Model file for the job. Use its own axes, mm. Give positions to 0.01 mm unless a question says otherwise; leave off trailing zeros. Write each loop counter-clockwise with the first axis right and the second up, starting at its lowest first coordinate (ties: lowest second). Pieces come first, ordered by that corner, then holes. Notation, with made-up numbers: (-35, 37) - (-28, 37) arc R22 ccw to (-28, 71) - close; hole circle Ø11 at (87, 53.25). An arc over 180 degrees is marked (long way). Use a Markdown table: item, result. Add a question column.
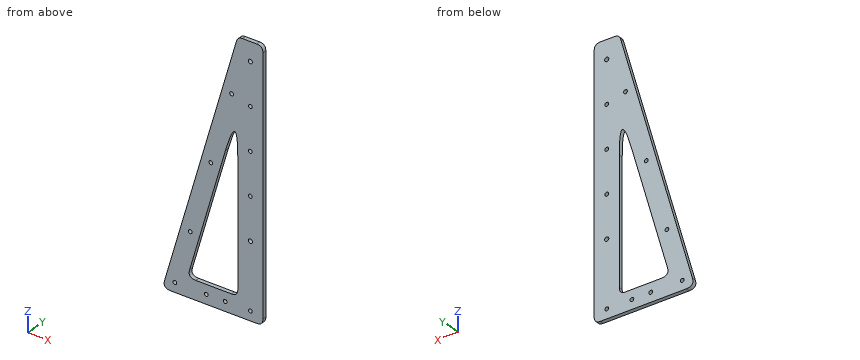
```python
from build123d import *

# Parameters (mm, degrees)
SKETCH1_R           = 1.5
SKETCH1_R_2         = 1.65
BOSS_EXTRUDE1_DEPTH = 3.175
FILLET1_SIZE        = 5


with BuildPart() as part:
    # Sketch1 → Boss-Extrude1 (new body)
    with BuildSketch(Plane(origin=(0, 0, 0), x_dir=(1, 0, 0), z_dir=(0, 1, 0))):
        Polygon((-20, -210), (0, -210), (0, 0), (-80, 0), align=None)
        with Locations(Location((-41.422797756, -107.71979577, 0), (0, 0, 270))):
            Circle(SKETCH1_R, mode=Mode.SUBTRACT)
        with Locations(Location((-24.939530082, -165.411232629, 0), (0, 0, 270))):
            Circle(SKETCH1_R, mode=Mode.SUBTRACT)
        with Locations(Location((-10, -195, 0), (0, 0, 270))):
            Circle(SKETCH1_R_2, mode=Mode.SUBTRACT)
        with BuildLine():
            ThreePointArc((-10, -159.75), (-8.5, -161.25), (-10, -162.75))
            ThreePointArc((-10, -162.75), (-11.5, -161.25), (-10, -159.75))
        make_face(mode=Mode.SUBTRACT)
        with BuildLine():
            ThreePointArc((-10, -126), (-8.5, -127.5), (-10, -129))
            ThreePointArc((-10, -129), (-11.5, -127.5), (-10, -126))
        make_face(mode=Mode.SUBTRACT)
        Polygon((-20, -15), (-20, -155.39917583), (-60.114050237, -15), align=None, mode=Mode.SUBTRACT)
        with Locations(Location((-57.90606543, -50.028358912, 0), (0, 0, 270))):
            Circle(SKETCH1_R, mode=Mode.SUBTRACT)
        with Locations(Location((-70.057025119, -7.5, 0), (0, 0, 270))):
            Circle(SKETCH1_R, mode=Mode.SUBTRACT)
        with Locations(Location((-45.028512559, -7.5, 0), (0, 0, 270))):
            Circle(SKETCH1_R, mode=Mode.SUBTRACT)
        with BuildLine():
            ThreePointArc((-10, -92.25), (-8.5, -93.75), (-10, -95.25))
            ThreePointArc((-10, -95.25), (-11.5, -93.75), (-10, -92.25))
        make_face(mode=Mode.SUBTRACT)
        with Locations(Location((-10, -60, 0), (0, 0, 270))):
            Circle(SKETCH1_R_2, mode=Mode.SUBTRACT)
        with Locations(Location((-30, -7.5, 0), (0, 0, 270))):
            Circle(SKETCH1_R, mode=Mode.SUBTRACT)
        with Locations(Location((-10, -7.5, 0), (0, 0, 270))):
            Circle(SKETCH1_R, mode=Mode.SUBTRACT)
    extrude(amount=BOSS_EXTRUDE1_DEPTH)

    # Fillet1
    # a fillet whose section is not a circle: 5 mm, written as the material it adds along each edge
    with BuildSketch(Plane(origin=(-20, 0, 15), x_dir=(0, 0, 1), z_dir=(0, 1, 0))) as fillet1_piece_1:
        with BuildLine():
            Bezier((FILLET1_SIZE, 0), (0, 0), (0, -FILLET1_SIZE), weights=[1, 1, 1])
            Line((0, -FILLET1_SIZE), (0, 0))
            Line((0, 0), (FILLET1_SIZE, 0))
        make_face()
    extrude(amount=3.175)
    with BuildSketch(Plane(origin=(-60.114050237, 0, 15), x_dir=(0.2747211278973786, 0, 0.9615239476408229), z_dir=(0, 1, 0))) as fillet1_piece_2:
        with BuildLine():
            Bezier((6.628649921, 0), (0, 0), (1.821030183, 6.373605639), weights=[1, 1, 1])
            Line((1.821030183, 6.373605639), (0, 0))
            Line((0, 0), (6.628649921, 0))
        make_face()
    extrude(amount=3.175)
    with BuildSketch(Plane(origin=(-20, 0, 155.39917583), x_dir=(-0.274721127897378, 0, -0.961523947640823), z_dir=(0, 1, 0))) as fillet1_piece_3:
        with BuildLine():
            Bezier((35.700274723, 0), (0, 0), (34.326669084, -9.807619738), weights=[1, 1, 1])
            Line((34.326669084, -9.807619738), (0, 0))
            Line((0, 0), (35.700274723, 0))
        make_face()
    extrude(amount=3.175)
    # a fillet whose section is not a circle: 5 mm, written as the material it takes off along each edge
    with BuildSketch(Plane(origin=(-80, -16.571624802, 0), x_dir=(0.2747211278973785, 0, 0.9615239476408229), z_dir=(0, 1, 0))) as fillet1_2_piece_1:
        with BuildLine():
            Bezier((6.628649921, 0), (0, 0), (1.821030183, 6.373605639), weights=[1, 1, 1])
            Line((1.821030183, 6.373605639), (0, 0))
            Line((0, 0), (6.628649921, 0))
        make_face()
    extrude(amount=36.318249605, mode=Mode.SUBTRACT)
    with BuildSketch(Plane(origin=(0, -12.5, 0), x_dir=(-1, 0, 0), z_dir=(0, 1, 0))) as fillet1_2_piece_2:
        with BuildLine():
            Bezier((FILLET1_SIZE, 0), (0, 0), (0, FILLET1_SIZE), weights=[1, 1, 1])
            Line((0, FILLET1_SIZE), (0, 0))
            Line((0, 0), (FILLET1_SIZE, 0))
        make_face()
    extrude(amount=28.175, mode=Mode.SUBTRACT)
    with BuildSketch(Plane(origin=(0, -12.5, 210), x_dir=(-1, 0, 0), z_dir=(0, 1, 0))) as fillet1_2_piece_3:
        with BuildLine():
            Bezier((FILLET1_SIZE, 0), (0, 0), (0, -FILLET1_SIZE), weights=[1, 1, 1])
            Line((0, -FILLET1_SIZE), (0, 0))
            Line((0, 0), (FILLET1_SIZE, 0))
        make_face()
    extrude(amount=28.175, mode=Mode.SUBTRACT)
    with BuildSketch(Plane(origin=(-20, -9.428767659, 210), x_dir=(-0.2747211278973768, 0, -0.9615239476408235), z_dir=(0, 1, 0))) as fillet1_2_piece_4:
        with BuildLine():
            Bezier((3.771507064, 0), (0, 0), (-1.036112674, -3.626394361), weights=[1, 1, 1])
            Line((-1.036112674, -3.626394361), (0, 0))
            Line((0, 0), (3.771507064, 0))
        make_face()
    extrude(amount=22.032535319, mode=Mode.SUBTRACT)


solid = part.part
```
(1) Flat gauge pins, fed straight in: pin 1 (1.5 mm diameter, centred on y = 1.5, z = 68, fed in from -X); pin 2 (1.6 mm diameter, centred on y = 2, z = 59, fed in from -X). Where does each tip first touch, or does it go through?
(2) Probe probe 1 along X at (y, z) = (0.55, 95); probe 2 along X at (y, z) = (1.15, 7.5); probe 3 along X at (y, z) = (1.55, 56). List the from-to ranges inside material, lowest first. Write a range as [from, to].
(3) Band-saw the part on D-D (y = 1.85). Give the number of separate pieces and of enclosed holes in the cut face, then the cut area to 3 significant figures.
(4) Band-saw the part on B-B (x = -37). Write the cut outline in (y, z) (3 decimals).
(5) Band-saw the part on A-A (z = 29.5). Write the cut outline in (x, y) (3 decimals), then the cut area to 3 significant figures.
(6) Band-saw the part on C-C (x = -64.5). Write the cut outline in (y, z) (3 decimals).
Model answer:
| question | item | result |
|---|---|---|
| 1 | pin 1 | stops at x = -60.79 |
| 1 | pin 2 | stops at x = -63.37 |
| 2 | probe 1 | x = [-52.86, -37.26], [-20, -10.83], [-9.17, 0] |
| 2 | probe 2 | x = [-77.86, -71.56], [-68.56, -46.53], [-43.53, -31.5], [-28.5, -11.5], [-8.5, 0] |
| 2 | probe 3 | x = [-64, -48.4], [-20, 0] |
| 3 | separate pieces | 1 |
| 3 | enclosed holes | 13 |
| 3 | area | 7,650 mm^2 |
| 4 | outline | (0, 0) - (3.175, 0) - (3.175, 15) - (0, 15) - close; (0, 95.899) - (3.175, 95.899) - (3.175, 150.5) - (0, 150.5) - close |
| 5 | outline | (-71.571, 0) - (-55.971, 0) - (-55.971, 3.175) - (-71.571, 3.175) - close; (-20, 0) - (0, 0) - (0, 3.175) - (-20, 3.175) - close |
| 5 | area | 113 mm^2 |
| 6 | outline | (0, 0) - (3.175, 0) - (3.175, 54.25) - (0, 54.25) - close |
